Part model, mm, in its own coordinate system. A direction names the side the tool comes from. Give positions to 0.01 mm unless a question says otherwise; leave off trailing zeros. Write each loop counter-clockwise with the first axis right and the second up, starting at its lowest first coordinate (ties: lowest second). Pieces come first, ordered by that corner, then holes. Notation, with made-up numbers: M 12.25,26.5 L 67.25,26.5 A18 cw 67.25,52.5 Z; hole C 88,-31 d8. An arc over 180 degrees is marked long. Answer as CSV lines item,"result". Start each with the question number.
Item 1: Pin check, flat tips, straight feed: pin 1 (6 mm diameter, centred on y = 21.5, z = 22, fed in from +X); pin 2 (7 mm diameter, centred on y = 0, z = 1.5, fed in from +X); pin 3 (5 mm diameter, centred on y = 4.5, z = -14, fed in from -X); pin 4 (2 mm diameter, centred on x = 125, z = -7, fed in from -Y). Stop position of each tip, or through.
Item 2: Two-plate mould, pull along Z, no slides. Class faces 1 (the cylindrical face through (156, 0, 6)), 2 (the flat face through (162, -3, 17)), 3 (the cylindrical face through (-141.13, -31.24, 6.94)): +Z half, -Z half, draft (parallel to the pull), parting line (faces both ways), or undercut.
Item 3: Band-saw the part on C-C, the plane x = 55.5. List the corners of the cut face in (y, z).
Item 4: Band-saw the part on D-D, the plane z = -18.5. List the corners of the cut face in (x, y), then the cut area to 3 significant figures.
Item 5: Band-saw the part on B-B, the plane y = -13. List the corners of the cut face in (x, z).
Item 6: Wall check: L1, parallel to Y at x = 156, z = 20; L2, parallel to X at y = -16, z = -16; L3, parallel to Y at x = -109.5, z = -4. Give the ranges that are in metal, low to high. Write a range as from..to.
Item 7: 3-axis set-ups, long thin cutter, end or side, ignore diameter. For faces 4 (the cylindrical face through (-157.07, -1.947, 2.539)), 5 (the cylindrical face through (-1.848, 30.736, 4.036)), 6 (the flat face through (162, -3, -3)), 7 (the cylindrical face through (140.87, -31.24, 6.94)), 8 (the flat face through (152, 0, 0)): which of +Z, -Z, +X, -X, +Y, -Y reach the whole face in a straight line?
Item 8: Band-saw the part on A-A, the plane z = 0. List the corners of the cut face in (x, y).
from build123d import *

# Parameters (mm, degrees)
BODY_START          = -150
SKETCH1_R           = 31
BODY_DEPTH          = 300
END_CAP_IN_START    = -150
SKETCH2_R           = 32
END_CAP_IN_DEPTH    = 18
END_CAP_OUT_START   = 132
SKETCH3_R           = 32
END_CAP_OUT_DEPTH   = 18
INLET_PORT_START    = -162
SKETCH4_R           = 6
INLET_PORT_DEPTH    = 12
INLET_SOCKET_START  = -162
SKETCH5_R           = 3.2
INLET_SOCKET_DEPTH  = 10
OUTLET_PORT_START   = 150
SKETCH6_R           = 6
OUTLET_PORT_DEPTH   = 12
OUTLET_SOCKET_START = 152
SKETCH7_R           = 3.2
OUTLET_SOCKET_DEPTH = 10
REJECT_PORT_START   = 150
SKETCH8_R           = 6
REJECT_PORT_DEPTH   = 12
REJECT_SOCKET_START = 162
SKETCH9_R           = 3.2
REJECT_SOCKET_DEPTH = 10


with BuildPart() as part:
    # Sketch1 → Body (new body)
    with BuildSketch(Plane(origin=(0, 0, 0), x_dir=(0, 0, -1), z_dir=(1, 0, 0)).offset(BODY_START)):
        Circle(SKETCH1_R)
    extrude(amount=BODY_DEPTH)

    # Sketch2 → End_Cap_In (add)
    with BuildSketch(Plane(origin=(0, 0, 0), x_dir=(0, 0, -1), z_dir=(1, 0, 0)).offset(END_CAP_IN_START)):
        Circle(SKETCH2_R)
    extrude(amount=END_CAP_IN_DEPTH)

    # Sketch3 → End_Cap_Out (add)
    with BuildSketch(Plane(origin=(0, 0, 0), x_dir=(0, 0, -1), z_dir=(1, 0, 0)).offset(END_CAP_OUT_START)):
        Circle(SKETCH3_R)
    extrude(amount=END_CAP_OUT_DEPTH)

    # Sketch4 → Inlet_Port (add)
    with BuildSketch(Plane(origin=(0, 0, 0), x_dir=(0, 0, -1), z_dir=(1, 0, 0)).offset(INLET_PORT_START)):
        Circle(SKETCH4_R)
    extrude(amount=INLET_PORT_DEPTH)

    # Sketch5 → Inlet_Socket (cut)
    with BuildSketch(Plane(origin=(0, 0, 0), x_dir=(0, 0, -1), z_dir=(1, 0, 0)).offset(INLET_SOCKET_START)):
        Circle(SKETCH5_R)
    extrude(amount=INLET_SOCKET_DEPTH, mode=Mode.SUBTRACT)

    # Sketch6 → Outlet_Port (add)
    with BuildSketch(Plane(origin=(0, 0, 0), x_dir=(0, 0, -1), z_dir=(1, 0, 0)).offset(OUTLET_PORT_START)):
        Circle(SKETCH6_R)
    extrude(amount=OUTLET_PORT_DEPTH)

    # Sketch7 → Outlet_Socket (cut)
    with BuildSketch(Plane(origin=(0, 0, 0), x_dir=(0, 0, -1), z_dir=(1, 0, 0)).offset(OUTLET_SOCKET_START)):
        Circle(SKETCH7_R)
    extrude(amount=OUTLET_SOCKET_DEPTH, mode=Mode.SUBTRACT)

    # Sketch8 → Reject_Port (add)
    with BuildSketch(Plane(origin=(0, 0, 0), x_dir=(0, 0, -1), z_dir=(1, 0, 0)).offset(REJECT_PORT_START)):
        with Locations((-20, 0)):
            Circle(SKETCH8_R)
    extrude(amount=REJECT_PORT_DEPTH)

    # Sketch9 → Reject_Socket (cut)
    with BuildSketch(Plane(origin=(0, 0, 0), x_dir=(0, 0, -1), z_dir=(1, 0, 0)).offset(REJECT_SOCKET_START)):
        with Locations((-20, 0)):
            Circle(SKETCH9_R)
    extrude(amount=-REJECT_SOCKET_DEPTH, mode=Mode.SUBTRACT)


solid = part.part
Output:
1,pin 1,"x = 150"
1,pin 2,"x = 162"
1,pin 3,"x = -150"
1,pin 4,"y = -30.41"
2,face 1,"undercut"
2,face 2,"draft"
2,face 3,"parting line"
3,outline,"C 0,0 d62"
4,outline,"M -150,-26.11 L -132,-26.11 L -132,-24.87 L 132,-24.87 L 132,-26.11 L 150,-26.11 L 150,26.11 L 132,26.11 L 132,24.87 L -132,24.87 L -132,26.11 L -150,26.11 Z"
4,area,"15,000 mm²"
5,outline,"M -150,-29.24 L -132,-29.24 L -132,-28.14 L 132,-28.14 L 132,-29.24 L 150,-29.24 L 150,29.24 L 132,29.24 L 132,28.14 L -132,28.14 L -132,29.24 L -150,29.24 Z"
6,L1,"-6..-3.2, 3.2..6"
6,L2,"-150..150"
6,L3,"-30.74..30.74"
7,face 4,"-X"
7,face 5,"none"
7,face 6,"+Z, -Z, +X, +Y, -Y"
7,face 7,"+X, -X"
7,face 8,"+X"
8,outline,"M -162,-6 L -150,-6 L -150,-32 L -132,-32 L -132,-31 L 132,-31 L 132,-32 L 150,-32 L 150,-6 L 162,-6 L 162,-3.2 L 152,-3.2 L 152,3.2 L 162,3.2 L 162,6 L 150,6 L 150,32 L 132,32 L 132,31 L -132,31 L -132,32 L -150,32 L -150,6 L -162,6 L -162,3.2 L -152,3.2 L -152,-3.2 L -162,-3.2 Z"
